from build123d import *

# Parameters (mm, degrees)
CROQUIS1_R              = 1.75
CROQUIS1_R_2            = 3.5
CROQUIS1_R_3            = 2
SALIENTE_EXTRUIR1_DEPTH = 3


with BuildPart() as part:
    # Croquis1 → Saliente-Extruir1 (new body)
    with BuildSketch(Plane(origin=(0, 0, 0), x_dir=(0, 0, -1), z_dir=(1, 0, 0))):
        with BuildLine():
            ThreePointArc((-12.479760771, -8.321993217), (10.178991806, -11.017627957), (9.281950646, 11.783267467))
            add(Edge.make_bspline(
                [(-153.589400871, 9.333606023), (-52.027464553, 57.017454048), (-3.028685523, 21.666117386), (9.281950646, 11.783267467)],
                knots=[0, 0, 0, 0, 1, 1, 1, 1], degree=3))
            ThreePointArc((-153.589400871, 9.333606023), (-158.998047864, -4.362927301), (-144.894564169, -8.598518767))
            add(Edge.make_bspline(
                [(-144.894564169, -8.598518767), (-94.399563679, 13.089335746), (-29.021790265, 9.608207487), (-12.479760771, -8.321993217)],
                knots=[0, 0, 0, 0, 1, 1, 1, 1], degree=3))
        make_face()
        with Locations((-150, 0)):
            Circle(CROQUIS1_R, mode=Mode.SUBTRACT)
        Circle(CROQUIS1_R_2, mode=Mode.SUBTRACT)
        with Locations((-113, 13.11718)):
            Circle(CROQUIS1_R_3, mode=Mode.SUBTRACT)
        with Locations((-30, 15.614781046)):
            Circle(CROQUIS1_R_3, mode=Mode.SUBTRACT)
    extrude(amount=SALIENTE_EXTRUIR1_DEPTH)


solid = part.part
The listing builds one solid part. Answer for the finished solid, in the listing's coordinates (mm). Give positions to 0.01 mm unless a question says otherwise; leave off trailing zeros.
Item 1: Flat-ended cylindrical pins translate along their axes: P1, Ø1.5, axis at x = 1, z = 108, coming from the -Y side; P2, Ø2, axis at y = 0, z = 150, coming from the +X side. Find the tip coordinate at first contact, or state that the pin passes through.
Item 2: Section A-A, the plane x = 0.5 is taken. Count the separate pieces of the cut face and the enclosed holes in it, plus the area to 3 significant figures.
Item 3: Find the intervals of material crossed by line 1 along Y through (x, z) = (1.7, 0); line 2 along Y through (x, z) = (1, 113); line 3 along Y through (x, z) = (2.5, 117), in increasing order.
Item 4: Determine the mould class of faces 1 (the cylindrical face through (1.5, 13.2, 115)), 2 (the cylindrical face through (1.48, -4.15, 159.1)), 3 (the cylindrical face through (1.479, 0.526, 148.331)), 4 (the flat face through (3, 16, 66)) for opening direction Y: released by +Y, released by -Y, zero draft, split by the parting line, or undercut.
Completed:
1. P1: stops at y = 2.45
1. P2: passes through
2. separate pieces: 1
2. enclosed holes: 4
2. area: 4,450 mm2
3. line 1: y = -15 to -3.5, 3.5 to 18.34
3. line 2: y = 1.55 to 11.12, 15.12 to 25.07
3. line 3: y = 0.62 to 23.84
4. face 1: undercut
4. face 2: split by the parting line
4. face 3: undercut
4. face 4: zero draft
